```python
from build123d import *

# Parameters (mm, degrees)
F2_DEPTH = 79.248
F0_W     = 25.4
F0_H     = 19.0499988828
F3_DEPTH = 25.4


with BuildPart() as f2:
    # F0 (on Front) → F2 (new body)
    with BuildSketch(Plane.XZ):
        Polygon((41.275, -9.525), (41.275, 9.525), (22.2250011172, 9.525), (-41.275, 9.525), (-41.275, -9.525), align=None)
        with BuildLine():
            Line((-41.275, 9.525), (22.2250011172, 9.525))
            Line((22.2250011172, 9.525), (22.2250011172, 27.0002))
            ThreePointArc((22.2250011172, 27.0002), (32.1759573239, 51.4143913521), (56.358301529, 61.9162244085))
            add(Edge.make_bspline(
                [(-41.275, 9.525), (-40.962193468, 30.2773661311), (10.7351419733, 61.2238694952), (56.358301529, 61.9162244085)],
                knots=[0, 0, 0, 0, 110.8627649737, 110.8627649737, 110.8627649737, 110.8627649737], degree=3))
        make_face()
    extrude(amount=F2_DEPTH)

    # F0 (on Front) → F3 (join)
    with BuildSketch(Plane.XZ):
        Polygon((41.275, -9.525), (41.275, 9.525), (22.2250011172, 9.525), (-41.275, 9.525), (-41.275, -9.525), align=None)
        with BuildLine():
            Line((22.2250011172, 9.525), (41.275, 9.525))
            Line((41.275, 9.525), (41.275, 27.0002))
            ThreePointArc((41.275, 27.0002), (45.9246798487, 38.2255201513), (57.15, 42.8752))
            Line((57.15, 42.8752), (60.325, 42.8752))
            Line((60.325, 42.8752), (60.325, 61.9251988828))
            Line((60.325, 61.9251988828), (57.15, 61.9251988828))
            add(Edge.make_bspline(
                [(56.358301529, 61.9162244085), (56.622408287, 61.9202323644), (56.8863114928, 61.9232264714), (57.15, 61.9251988828)],
                knots=[110.8627649737, 110.8627649737, 110.8627649737, 110.8627649737, 111.5045356385, 111.5045356385, 111.5045356385, 111.5045356385], degree=3))
            ThreePointArc((56.358301529, 61.9162244085), (32.1759573239, 51.4143913521), (22.2250011172, 27.0002))
            Line((22.2250011172, 27.0002), (22.2250011172, 9.525))
        make_face()
        with BuildLine():
            Line((-41.275, 9.525), (22.2250011172, 9.525))
            Line((22.2250011172, 9.525), (22.2250011172, 27.0002))
            ThreePointArc((22.2250011172, 27.0002), (32.1759573239, 51.4143913521), (56.358301529, 61.9162244085))
            add(Edge.make_bspline(
                [(-41.275, 9.525), (-40.962193468, 30.2773661311), (10.7351419733, 61.2238694952), (56.358301529, 61.9162244085)],
                knots=[0, 0, 0, 0, 110.8627649737, 110.8627649737, 110.8627649737, 110.8627649737], degree=3))
        make_face()
        with BuildLine():
            ThreePointArc((57.15, 61.9251988828), (56.7541253323, 61.9229551922), (56.358301529, 61.9162244085))
            add(Edge.make_bspline(
                [(56.358301529, 61.9162244085), (56.622408287, 61.9202323644), (56.8863114928, 61.9232264714), (57.15, 61.9251988828)],
                knots=[110.8627649737, 110.8627649737, 110.8627649737, 110.8627649737, 111.5045356385, 111.5045356385, 111.5045356385, 111.5045356385], degree=3))
        make_face()
        Polygon((85.725, 42.8752), (60.325, 42.8752), (60.325, 38.1), (111.125, 38.1), (111.125, 66.675), (60.325, 66.675), (60.325, 61.9251988828), (85.725, 61.9251988828), align=None)
        with Locations((73.025, 52.4001994414)):
            Rectangle(F0_W, F0_H)
    extrude(amount=F3_DEPTH)


solid = f2.part
```
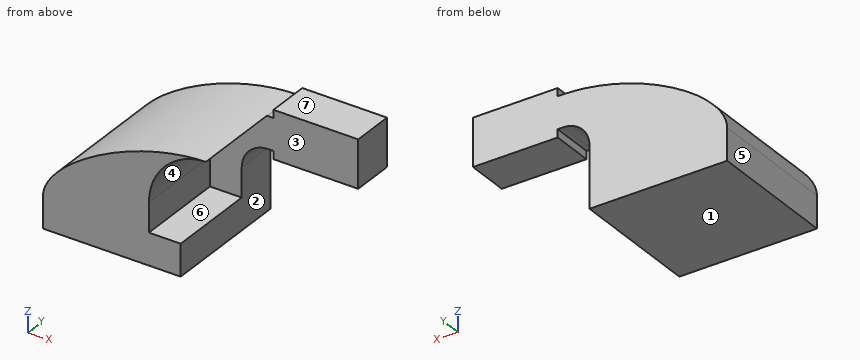
Source: CAD feature listing. Evaluate the final solid. Frame: model axes, mm. Face numbers are marked on the shaded views. A direction names the side the tool comes from. Round coordinates to 2 decimals unless told otherwise and drop trailing zeros. Write each loop counter-clockwise with the first axis right and the second up, starting at its lowest first coordinate (ties: lowest second). Pieces come first, ordered by that corner, then holes. Notation, with made-up numbers: M 19.5,-7 L 70.5,-7 A33 cw 70.5,28 Z; hole C 74,53 d4. An arc over 180 degrees is marked long. Answer as a JSON object with one key per item and string values. Group by question number.
(1) Section query A-A on x = 97. Output: boundary loops of the cut face in (y, z) (3 decimals), then the cut area to 3 significant figures.
(2) Mould query, pull axis Z, two halves, no side actions, for the marked faces 4, 5, 6 and 7. Classes: +Z half, -Z half, draft (parallel to the pull), parting line (faces both ways), or undercut.
(3) Ray query, line 1 (Y direction, x = 94, z = 42); line 2 (Z direction, x = 92.5, y = -17.5) (3 decimals); line 3 (X direction, y = -69, z = 1) (3 decimals). Return the intervals inside material, ascending. Write a range as [from, to].
(4) Section query B-B on z = -5. Output: boundary loops of the cut face in (x, y) (3 decimals), then the cut area to 3 significant figures.
(5) First-contact query: pin 1 (12.5 mm diameter, centred on x = 89.5, y = -9.5, fed in from -Z); pin 2 (18.5 mm diameter, centred on y = -26, z = 6.5, fed in from +X) (3 decimals); pin 3 (12 mm diameter, centred on x = 23, y = -54, fed in from +Z). Flat tips, straight axial feed; report the tip coordinate or a pass-through.
(6) Reachability of the marked faces 1, 2 and 3 from +Z, -Z, +X, -X, +Y, -Y: full face, straight path, thin tool, end or side. Return the list, or none.
Computed values:
{
 "1": {"outline": "M -25.4,38.1 L 0,38.1 L 0,66.675 L -25.4,66.675 Z", "area": "726 mm^2"},
 "2": {"face 4": "undercut", "face 5": "draft", "face 6": "undercut", "face 7": "+Z half"},
 "3": {"line 1": "[-25.4, 0]", "line 2": "[38.1, 66.675]", "line 3": "[-41.275, 41.275]"},
 "4": {"outline": "M -41.275,-79.248 L 41.275,-79.248 L 41.275,0 L -41.275,0 Z", "area": "6,540 mm^2"},
 "5": {"pin 1": "z = 38.1", "pin 2": "x = 41.275", "pin 3": "z = 58.26"},
 "6": {"face 1": "-Z, +X, -X, +Y, -Y", "face 2": "-Z, +X, +Y, -Y", "face 3": "+X, -Y"}
}
